```python
from build123d import *

# Parameters (mm, degrees)
BOSS_EXTRUDE1_DEPTH = 5
BOSS_EXTRUDE2_DEPTH = 15
SKETCH3_W           = 5
SKETCH3_H           = 35
BOSS_EXTRUDE3_DEPTH = 15
SKETCH4_W           = 5
SKETCH4_H           = 35
BOSS_EXTRUDE4_DEPTH = 5
BOSS_EXTRUDE5_DEPTH = 5
SKETCH7_R           = 1.8
CUT_EXTRUDE1_DEPTH  = 6


with BuildPart() as part:
    # Sketch1 → Boss-Extrude1 (new body)
    with BuildSketch(Plane.XY):
        Polygon((-7.529880478, -25.806772908), (27.470119522, -25.806772908), (27.470119522, -10.806772908), (7.470119522, -10.806772908), (7.470119522, 9.193227092), (-7.529880478, 9.193227092), align=None)
    extrude(amount=BOSS_EXTRUDE1_DEPTH)



with BuildPart() as body_2:
    # Sketch2 → Boss-Extrude2 (new body)
    with BuildSketch(Plane(origin=(0, 0, 0), x_dir=(-1, 0, 0), z_dir=(0, 0, -1))):
        Polygon((-7.470119522, 9.193227092), (-12.470119522, 9.193227092), (-12.470119522, -5.806772908), (-27.470119522, -5.806772908), (-27.470119522, -10.806772908), (-7.470119522, -10.806772908), align=None)
    extrude(amount=BOSS_EXTRUDE2_DEPTH)


with BuildPart() as body_3:
    # Sketch3 → Boss-Extrude3 (new body)
    with BuildSketch(Plane(origin=(0, 0, 0), x_dir=(-1, 0, 0), z_dir=(0, 0, -1))):
        with Locations((10.029880478, -8.306772908)):
            Rectangle(SKETCH3_W, SKETCH3_H)
    extrude(amount=BOSS_EXTRUDE3_DEPTH)


with BuildPart() as part_1:
    add(part.part)

    add(body_3.part)  # Boss-Extrude4 merges body 3
    # Sketch4 → Boss-Extrude4 (add)
    with BuildSketch(Plane.XY):
        with Locations((-10.029880478, -8.306772908)):
            Rectangle(SKETCH4_W, SKETCH4_H)
    extrude(amount=BOSS_EXTRUDE4_DEPTH)


    add(body_2.part)  # Boss-Extrude5 merges body 2
    # Sketch5 → Boss-Extrude5 (add)
    with BuildSketch(Plane.XY):
        Polygon((7.470119522, 9.193227092), (7.470119522, -10.806772908), (27.470119522, -10.806772908), (27.470119522, -5.806772908), (12.470119522, -5.806772908), (12.470119522, 9.193227092), align=None)
    extrude(amount=BOSS_EXTRUDE5_DEPTH)

    # Sketch7 → Cut-Extrude1 (cut, through all)
    with BuildSketch(Plane(origin=(0, 0, 0), x_dir=(-1, 0, 0), z_dir=(0, 0, -1))):
        with Locations((0.029880478, 1.693227092)):
            Circle(SKETCH7_R)
        with Locations((-17.470119522, -18.306772908)):
            Circle(SKETCH7_R)
    extrude(amount=-CUT_EXTRUDE1_DEPTH, mode=Mode.SUBTRACT)


solid = part_1.part
```
Model file for the job. Use its own axes, mm. A direction names the side the tool comes from. Coordinates: 2 decimals unless noted, no trailing zeros. Loops run counter-clockwise (first coordinate to the right, second up) from the corner with the lowest first, then second, coordinate; pieces in that order, holes last. Notation, with made-up numbers: (-38.5, 62.25) - (-15.5, 62.25) arc R10 cw to (-15.5, 67.25) - close; hole circle Ø7 at (62, -24.75). An arc over 180 degrees is marked (long way). Answer as a JSON object with one key per item and string values. Group by question number.
(1) Cut at A-A (z = -11). Give the cut face in (x, y), then the cut area to 3 significant figures.
(2) Cut at B-B (y = -17). Give the cut face in (x, z), then the cut area to 3 significant figures.
(3) Cut at D-D (y = -2). Give the cut face in (x, z).
(4) Two-plate mould, pull along X, no slides. Class faces 4 (the face through (12.47, 2, -5)), 5 (the face through (18, -10.807, -7)), 6 (the face through (-7.53, -9, -7)): released by +X, released by -X, zero draft, split by the parting line, or undercut.
(5) Flat gauge pins, fed straight in: pin 1 (2 mm diameter, centred on x = 17.47, y = -18.31, fed in from -Z); pin 2 (4.5 mm diameter, centred on x = 21.5, z = 0, fed in from +Y); pin 3 (7.5 mm diameter, centred on y = -16, z = -10.5, fed in from +X); pin 4 (4.5 mm diameter, centred on x = -0.03, y = 1.69, fed in from -Z). Where does each tip first touch, or does it go through?
(6) Tool access for faces 1 (the face through (20, -5.807, -5)), 2 (the face through (-10, -8, -15)), 3 (the face through (7.47, -1, -7)): list every direction of +Z, -Z, +X, -X, +Y, -Y with a clear straight run to the whole face (end or side of a thin tool).
(7) Probe line 1 along X through (y, z) = (1, -1.5); line 2 along X through (y, z) = (-10, -6); line 3 along Z through (x, y) = (-1, -10.5). List the from-to ranges inside material, lowest first.
(8) Cut at C-C (x = 14). Give the cut face in (y, z).
Geometry says:
{
 "1": {"outline": "(-12.53, -25.81) - (-7.53, -25.81) - (-7.53, 9.19) - (-12.53, 9.19) - close; (7.47, -10.81) - (27.47, -10.81) - (27.47, -5.81) - (12.47, -5.81) - (12.47, 9.19) - (7.47, 9.19) - close", "area": "350 mm^2"},
 "2": {"outline": "(-12.53, -15) - (-7.53, -15) - (-7.53, 0) - (16.23, 0) - (16.23, 5) - (-12.53, 5) - close; (18.71, 0) - (27.47, 0) - (27.47, 5) - (18.71, 5) - close", "area": "263 mm^2"},
 "3": {"outline": "(-12.53, -15) - (-7.53, -15) - (-7.53, 0) - (7.47, 0) - (7.47, -15) - (12.47, -15) - (12.47, 5) - (-12.53, 5) - close"},
 "4": {"face 4": "released by +X", "face 5": "zero draft", "face 6": "undercut"},
 "5": {"pin 1": "passes through", "pin 2": "stops at y = -5.81", "pin 3": "stops at x = -7.53", "pin 4": "stops at z = 0"},
 "6": {"face 1": "+Z, -Z, +X, +Y", "face 2": "-Z, +X, -X, +Y, -Y", "face 3": "-Z, +Y, -Y"},
 "7": {"line 1": "x = -12.53 to -7.53, 7.47 to 12.47", "line 2": "x = -12.53 to -7.53, 7.47 to 27.47", "line 3": "z = 0 to 5"},
 "8": {"outline": "(-25.81, 0) - (-10.81, 0) - (-10.81, -15) - (-5.81, -15) - (-5.81, 5) - (-25.81, 5) - close"}
}
